Geometry: see drawing. Coordinates: mm, zero at the bounding-box minimum. A direction names the side the tool comes from. Round coordinates to 2 decimals unless told otherwise and drop trailing zeros. Loops run counter-clockwise (first coordinate to the right, second up) from the corner with the lowest first, then second, coordinate; pieces in that order, holes last. Notation, with made-up numbers: M 56,60.5 L 69,60.5 A19 cw 69,82.5 Z; hole C 68.5,13.5 d4. An arc over 180 degrees is marked long. Answer as a JSON object with one key per item and string values.
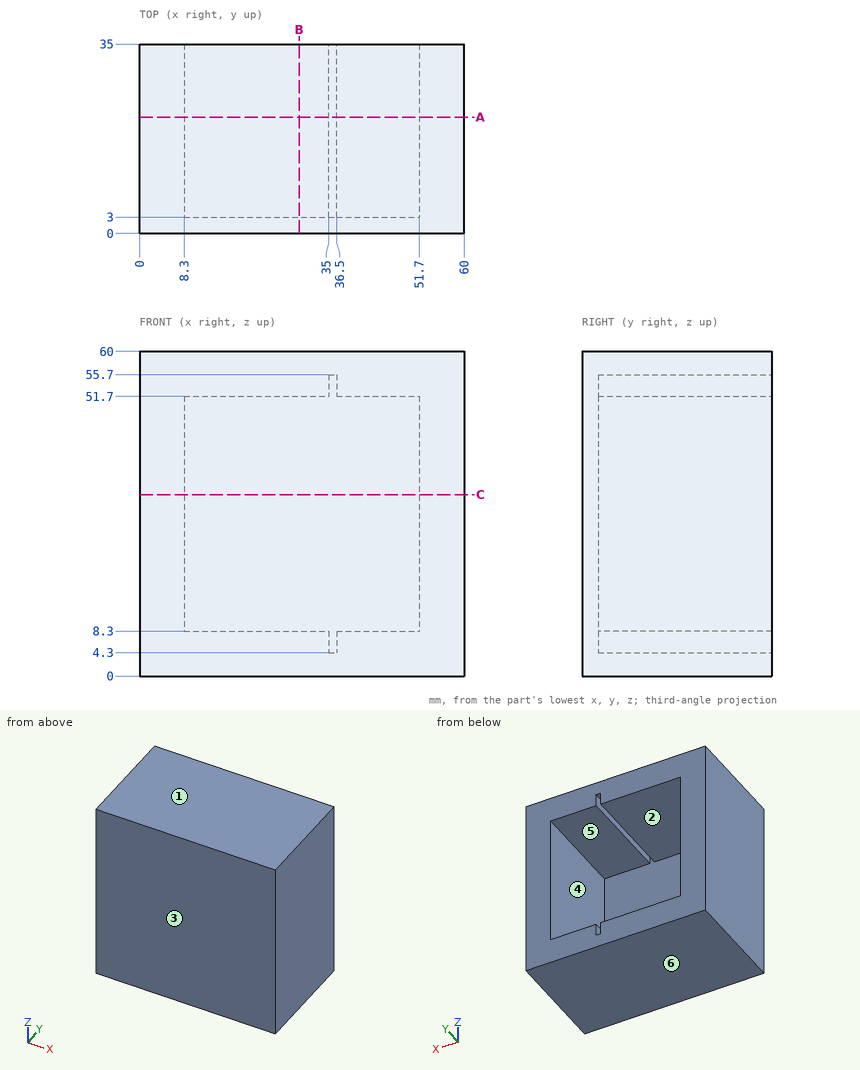
1) Section query B-B (x = 29.5). Return the cut outline in (y, z).
Results:
{"outline": "M 0,0 L 35,0 L 35,8.3 L 3,8.3 L 3,51.7 L 35,51.7 L 35,60 L 0,60 Z"}
2) Section query C-C (z = 33.5). Return the cut outline in (x, y), and give its area (3 significant figures).
Results:
{"outline": "M 0,0 L 60,0 L 60,35 L 51.7,35 L 51.7,3 L 8.3,3 L 8.3,35 L 0,35 Z", "area": "711 mm2"}
3) Reachability of the marked faces 1 and 2 from +Z, -Z, +X, -X, +Y, -Y: full face, straight path, thin tool, end or side. Return the list, or none.
Results:
{"face 1": "+Z, +X, -X, +Y, -Y", "face 2": "+Y"}
4) Ray query, line 1 (X direction, y = 29, z = 38); line 2 (X direction, y = 30, z = 6.5). Return the intervals inside material, ascending.
Results:
{"line 1": "0 to 8.3, 51.7 to 60", "line 2": "0 to 35, 36.5 to 60"}
5) Section query A-A (y = 21.5). Return the cut outline in (x, z), and give its area (3 significant figures).
Results:
{"outline": "M 0,0 L 60,0 L 60,60 L 0,60 Z; hole M 8.3,8.3 L 35,8.3 L 35,4.3 L 36.5,4.3 L 36.5,8.3 L 51.7,8.3 L 51.7,51.7 L 36.5,51.7 L 36.5,55.7 L 35,55.7 L 35,51.7 L 8.3,51.7 Z", "area": "1,700 mm2"}
6) Pull-direction query (Z, two-part tool) for the marked faces 3, 4, 5 and 6; classes: +Z half, -Z half, draft (parallel to the pull), parting line (faces both ways), or undercut.
Results:
{"face 3": "draft", "face 4": "undercut", "face 5": "undercut", "face 6": "-Z half"}
